Geometry check sheet. Reference: the model listing, model coordinates, mm. Face numbers are marked on the shaded views. A direction names the side the tool comes from. Give positions to 0.01 mm unless a question says otherwise; leave off trailing zeros. Write each loop counter-clockwise with the first axis right and the second up, starting at its lowest first coordinate (ties: lowest second). Pieces come first, ordered by that corner, then holes. Notation, with made-up numbers: (80, 22.25) - (126, 22.25) arc R21 cw to (126, 38.25) - close; hole circle Ø4 at (-19, 54.25). An arc over 180 degrees is marked (long way). One line per question, with ' | ' between items. Start each with the question number.
Q1. Gauge pin test, flat ends, axial feed: P1, Ø2, axis at y = 24, z = 1.5, coming from the -X side; P2, Ø5, axis at x = -1.5, z = 2.5, coming from the -Y side; P3, Ø6, axis at x = 21, z = 8.5, coming from the +Y side; P4, Ø20.5, axis at x = 0, y = 0, coming from the -Z side. Record the tip position at first contact, or that the pin passes through.
Q2. Section check C-C on z = 3.25. Record the boundary of the cut face in (x, y), and give its area (3 significant figures).
Q3. Section check B-B on x = 0. Count the separate pieces of the cut face and the enclosed holes in it, and give its area (3 significant figures).
Q4. Release check for a two-part mould opening along Y. For the marked faces 3, 4, 5 and 6 record: +Y half, -Y half, draft (parallel to the pull), parting line (faces both ways), or undercut.
Q5. Section check D-D on z = 10.75. Record the boundary of the cut face in (x, y), and give its area (3 significant figures).
Q6. Set-up check for the marked faces 1 and 2: record each of +Z, -Z, +X, -X, +Y, -Y from which the full face is reachable in a straight line by a thin tool's end or side.
Q7. Thickness scan on L1, parallel to Y at x = 0, z = 8.75; L2, parallel to X at y = 26, z = 0.5; L3, parallel to Y at x = -23, z = 12. Record the ranges inside material, lowest first. Write a range as [from, to].
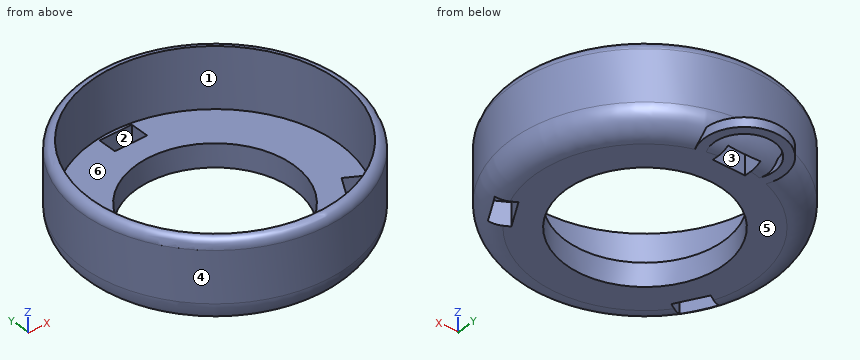
```python
from build123d import *

# Parameters (mm, degrees)
F0_R     = 28.7
F0_R_2   = 26.7
F1_DEPTH = 18
F2_R     = 26.7
F3_DEPTH = 13
F4_R     = 17
F4_W     = 7
F4_H     = 4
F5_DEPTH = 5.001
F7_R     = 1.99999
F8_R     = 8.5
F8_R_2   = 6.5
F9_DEPTH = 2


# Not quite as in the source:
# - a fillet or chamfer that OpenCascade refuses, or shapes differently, is made with other operations: its cross-section is extruded or revolved along the edge and cut away or added
# - a fillet or chamfer is up to 0.001 mm smaller than in the source, because OpenCascade refuses the exact size


with BuildPart() as f1:
    # F0 (on Top) → F1 (new body)
    with BuildSketch(Plane.XY):
        Circle(F0_R)
        Circle(F0_R_2, mode=Mode.SUBTRACT)
        Circle(F0_R_2)
    extrude(amount=F1_DEPTH)

    # F2 (on face) → F3 (cut)
    with BuildSketch(Plane.XY.offset(18)):
        Circle(F2_R)
    extrude(amount=-F3_DEPTH, mode=Mode.SUBTRACT)

    # F4 (on face) → F5 (cut, through all)
    with BuildSketch(Plane.XY.offset(5)):
        Circle(F4_R)
        with Locations((0, 24)):
            Rectangle(F4_W, F4_H)
        Polygon((-20.8025588833, -7.9689110868), (-24.2666604984, -9.9689110868), (-20.7666604984, -16.0310889132), (-17.3025588833, -14.0310889132), align=None)
        Polygon((17.3025588833, -14.0310889132), (20.7666604984, -16.0310889132), (24.2666604984, -9.9689110868), (20.8025588833, -7.9689110868), align=None)
    extrude(amount=-F5_DEPTH, mode=Mode.SUBTRACT)

    # F6: fillet of radius 5 on 1 edges, made by hand

    # F6_s1 → F6_t2 (revolve, cut)
    with BuildSketch(Plane.XZ):
        with BuildLine():
            ThreePointArc((28.7, 5), (27.2355339059, 1.4644660941), (23.7, 0))
            Line((23.7, 0), (28.7, 0))
            Line((28.7, 0), (28.7, 5))
        make_face()
    revolve(axis=Axis((0, 0, 0), (0, 0, 1)), mode=Mode.SUBTRACT)

    # F7 (radius 2 in the source; OpenCascade refuses exactly that, so slightly less here)
    f7_edges = [f1.edges().sort_by_distance(p)[0] for p in [
        (-28.7, 0, 18),
    ]]
    fillet(f7_edges, radius=F7_R)

    # F8 (on Top) → F9 (join)
    with BuildSketch(Plane.XY):
        with Locations((0, 26)):
            Circle(F8_R)
        with Locations((0, 26)):
            Circle(F8_R_2, mode=Mode.SUBTRACT)
    extrude(amount=F9_DEPTH)


solid = f1.part
```
Working result:
1) P1: stops at x = -15.27 | P2: stops at y = -28.69 | P3: stops at y = 22.35 | P4: passes through
2) outline: circle Ø56.77 at (0, 0); hole (-24.27, -9.97) - (-20.77, -16.03) - (-17.3, -14.03) - (-20.8, -7.97) - close; hole circle Ø34 at (0, 0); hole (-3.5, 22) - (3.5, 22) - (3.5, 26) - (-3.5, 26) - close; hole (17.3, -14.03) - (20.77, -16.03) - (24.27, -9.97) - (20.8, -7.97) - close | area: 1,540 mm2
3) separate pieces: 4 | enclosed holes: 0 | area: 141 mm2
4) face 3: undercut | face 4: parting line | face 5: draft | face 6: undercut
5) outline: circle Ø57.4 at (0, 0); hole circle Ø53.4 at (0, 0) | area: 348 mm2
6) face 1: +Z | face 2: +Z, -Z
7) L1: y = [-28.7, -26.7], [26.7, 28.7] | L2: x = [-8.5, -6.5], [6.5, 8.5] | L3: y = [-17.17, -13.56], [13.56, 17.17]
